```python
from build123d import *

# Parameters (mm, degrees)
F0_W     = 63.5
F0_H     = 63.5
F1_DEPTH = 1219.2
F2_W     = 63.5
F2_H     = 64.3730163574
F3_DEPTH = 63.5
F5_DEPTH = 76.2


with BuildPart() as f1:
    # F0 (on Front) → F1 (new body)
    with BuildSketch(Plane.XZ):
        with Locations((-86.9832811058, 6.737372756)):
            Rectangle(F0_W, F0_H)
    extrude(amount=F1_DEPTH)

    # F2 (on face) → F3 (join)
    with BuildSketch(Plane(origin=(0, 0, -25.012627244), x_dir=(1, 0, 0), z_dir=(0, 0, -1))):
        with Locations((-86.9832811058, 32.1865081787)):
            Rectangle(F2_W, F2_H)
    extrude(amount=F3_DEPTH)

    # F4 (on face) → F5 (cut)
    with BuildSketch(Plane(origin=(-118.7332811058, 0, 0), x_dir=(0, -1, 0), z_dir=(-1, 0, 0))):
        with BuildLine():
            Line((32.457142012, -49.1428072748), (32.3523825242, -64.3824472132))
            ThreePointArc((32.3523825242, -64.3824472132), (37.7743649699, -62.1692682367), (40.0247622681, -56.762627244))
            ThreePointArc((40.0247622681, -56.762627244), (37.8114032608, -51.3930245421), (32.457142012, -49.1428072748))
        make_face()
        with BuildLine():
            ThreePointArc((32.457142012, -49.1428072748), (24.7849422989, -56.7102475001), (32.3523825242, -64.3824472132))
            Line((32.3523825242, -64.3824472132), (32.457142012, -49.1428072748))
        make_face()
    extrude(amount=-F5_DEPTH, mode=Mode.SUBTRACT)


solid = f1.part
```
For this review, take the finished solid that the model builds, in its own axes (mm). A direction names the side the tool comes from. Round coordinates to 2 decimals unless told otherwise and drop trailing zeros. Loops run counter-clockwise (first coordinate to the right, second up) from the corner with the lowest first, then second, coordinate; pieces in that order, holes last.
Q1. To check wall thickness, follow line 1 along Y through (x, z) = (-68, -46); line 2 along Z through (x, y) = (-115, -78); line 3 along Y through (x, z) = (-111.5, -62). State the ranges of each line that lie inside material, in increasing order.
Result sheet:
line 1: y = -64.37 to 0
line 2: z = -25.01 to 38.49
line 3: y = -64.37 to -37.94, -26.87 to 0
Q2. Machinability: for faces 1 (the face through (-87, -634, -25.013)), 2 (the face through (-87, -1219.2, 7)), which of the approach directions +Z, -Z, +X, -X, +Y, -Y give a long, thin tool a straight path to every point of the face, cutting with its end or side? Answer none if there is none.
Result sheet:
face 1: -Z, +X, -X, -Y
face 2: +Z, -Z, +X, -X, -Y
Q3. Add section A-A on x = -80. Write out the cut boundary in (y, z), plus the area to 3 significant figures.
Result sheet:
outline: (-1219.2, -25.01) - (-64.37, -25.01) - (-64.37, -88.51) - (0, -88.51) - (0, 38.49) - (-1219.2, 38.49) - close; hole circle Ø15.24 at (-32.4, -56.76)
area: 81,300 mm2
Q4. Mouldability with a two-part tool opening along X and no side actions: class faces 3 (the face through (-87, -64.373, -56)), 4 (the face through (-118.733, -601, 4)), 5 (the face through (-55.233, -601, 4)) as +X half, -X half, draft (parallel to the pull), parting line (faces both ways), or undercut.
Result sheet:
face 3: draft
face 4: -X half
face 5: +X half
Q5. Insertion check: pin 1 Ø5 at (x, y) = (-97, -808) entering from -Z. The pin has a flat end and moves straight along its axis. Give the tip position at first contact, or say it passes through.
Result sheet:
pin 1: stops at z = -25.01
Q6. Add section B-B on y = -656.5. Write out the cut boundary in (x, z).
Result sheet:
outline: (-118.73, -25.01) - (-55.23, -25.01) - (-55.23, 38.49) - (-118.73, 38.49) - close
